from build123d import *

# Parameters (mm, degrees)
SKETCH1_R           = 2.25
BOSS_EXTRUDE1_DEPTH = 10
SKETCH2_R           = 12.2
CUT_EXTRUDE3_DEPTH  = 11
CHAMFER1_SIZE       = 0.5


with BuildPart() as part:
    # Sketch1 → Boss-Extrude1 (new body)
    with BuildSketch(Plane.XY):
        with BuildLine():
            Line((-13.228756555, 15), (13.228756555, 15))
            ThreePointArc((13.228756555, 15), (14.142135624, 14.142135624), (15, 13.228756555))
            Line((15, 13.228756555), (15, -13.228756555))
            ThreePointArc((15, -13.228756555), (14.142135624, -14.142135624), (13.228756555, -15))
            Line((13.228756555, -15), (-13.228756555, -15))
            ThreePointArc((-13.228756555, -15), (-14.142135624, -14.142135624), (-15, -13.228756555))
            Line((-15, -13.228756555), (-15, 13.228756555))
            ThreePointArc((-15, 13.228756555), (-14.142135624, 14.142135624), (-13.228756555, 15))
        make_face()
        with Locations((-11.313708499, 11.313708499)):
            Circle(SKETCH1_R, mode=Mode.SUBTRACT)
        with Locations((11.313708499, 11.313708499)):
            Circle(SKETCH1_R, mode=Mode.SUBTRACT)
        with Locations((11.313708499, -11.313708499)):
            Circle(SKETCH1_R, mode=Mode.SUBTRACT)
        with Locations((-11.313708499, -11.313708499)):
            Circle(SKETCH1_R, mode=Mode.SUBTRACT)
    extrude(amount=BOSS_EXTRUDE1_DEPTH)

    # Sketch2 → Cut-Extrude3 (cut, through all)
    with BuildSketch(Plane.XY.offset(10)):
        Circle(SKETCH2_R)
    extrude(amount=-CUT_EXTRUDE3_DEPTH, mode=Mode.SUBTRACT)

    # Chamfer1
    chamfer1_edges = [part.edges().sort_by_distance(p)[0] for p in [
        (-14.142135624, -14.142135624, 10),
        (-15, 0, 0),
        (-14.142135624, 14.142135624, 0),
        (0, -15, 10),
        (14.142135624, -14.142135624, 10),
        (15, 0, 10),
        (-13.563708499, 11.313708499, 0),
        (-13.563708499, 11.313708499, 10),
        (14.142135624, 14.142135624, 10),
        (9.063708499, 11.313708499, 0),
        (9.063708499, 11.313708499, 10),
        (0, 15, 10),
        (9.063708499, -11.313708499, 0),
        (9.063708499, -11.313708499, 10),
        (-13.563708499, -11.313708499, 0),
        (-13.563708499, -11.313708499, 10),
        (-14.142135624, 14.142135624, 10),
        (-12.2, 0, 0),
        (-12.2, 0, 10),
        (-15, 0, 10),
        (0, 15, 0),
        (14.142135624, 14.142135624, 0),
        (15, 0, 0),
        (14.142135624, -14.142135624, 0),
        (0, -15, 0),
        (-14.142135624, -14.142135624, 0),
    ]]
    chamfer(chamfer1_edges, length=CHAMFER1_SIZE)


solid = part.part
CAD build for the part. Positions are in the model's coordinates, mm. Round coordinates to 2 decimals unless told otherwise and drop trailing zeros. Loops run counter-clockwise (first coordinate to the right, second up) from the corner with the lowest first, then second, coordinate; pieces in that order, holes last. Notation, with made-up numbers: M 63.5,43 L 107.5,43 A18 cw 107.5,66 Z; hole C -3,86 d6. An arc over 180 degrees is marked long. One line per question, with ' | ' between items. Start each with the question number.
Item 1: Cut at A-A, the plane y = 0. Write the cut outline in (x, z), plus the area to 3 significant figures.
Item 2: Cut at C-C, the plane z = 6.5. Write the cut outline in (x, y).
Item 3: Two-plate mould, pull along X, no slides. Class faces 1 (the cylindrical face through (-10.1, 13.21, 4.94)), 2 (the conical face through (14, -14, 9.7)), 3 (the conical face through (-13.98, 13.95, 9.75)): pulls with the +X half, pulls with the -X half, needs draft (parallel to the pull), parting line crosses it, or undercut.
Item 4: Wall check: line 1 (Y direction, x = 0, z = 7.5); line 2 (Y direction, x = 10, z = 5.25); line 3 (Y direction, x = -11, z = 2.5). Give the ranges that are in metal, low to high.
Responses:
1) outline: M -15,0.5 L -14.5,0 L -12.7,0 L -12.2,0.5 L -12.2,9.5 L -12.7,10 L -14.5,10 L -15,9.5 Z; M 12.2,0.5 L 12.7,0 L 14.5,0 L 15,0.5 L 15,9.5 L 14.5,10 L 12.7,10 L 12.2,9.5 Z | area: 55.0 mm²
2) outline: M -15,-13.23 A20 ccw -13.23,-15 L 13.23,-15 A20 ccw 15,-13.23 L 15,13.23 A20 ccw 13.23,15 L -13.23,15 A20 ccw -15,13.23 Z; hole C -11.31,-11.31 d4.5; hole C -11.31,11.31 d4.5; hole C 0,0 d24.4; hole C 11.31,-11.31 d4.5; hole C 11.31,11.31 d4.5
3) face 1: undercut | face 2: pulls with the +X half | face 3: pulls with the -X half
4) line 1: y = -15 to -12.2, 12.2 to 15 | line 2: y = -15 to -13.14, -9.49 to -6.99, 6.99 to 9.49, 13.14 to 15 | line 3: y = -15 to -13.54, -9.09 to -5.28, 5.28 to 9.09, 13.54 to 15
